Here's how the part is built. I have some questions about the finished solid (model axes, mm). A direction names the side the tool comes from. Give positions to 0.01 mm unless a question says otherwise; leave off trailing zeros. Loops run counter-clockwise (first coordinate to the right, second up) from the corner with the lowest first, then second, coordinate; pieces in that order, holes last. Notation, with made-up numbers: (71.5, 49.5) - (81.5, 49.5) arc R31 cw to (81.5, 86.5) - close; hole circle Ø1 at (-1.5, 14). An arc over 180 degrees is marked (long way). Return JSON: item names as keys, results as strings. Group by question number.
(1) If we section it at D-D (z = -9): Please give me the cut outline in (x, y).
(2) For P1, Ø5.5, axis at x = 7.5, z = -23, coming from the +Y side; P2, Ø6.5, axis at y = 5.5, z = -20.5, coming from the +X side; P3, Ø3, axis at x = 11, z = -17, coming from the -Y side; P4, Ø8, axis at x = 9, z = 15.5, coming from the -Y side, each with a flat end and sliding along its axis, tell me the tip position at first contact or that it passes through.
(3) On a 3-axis mill with a long thin cutter (end or side, diameter ignored), from which of +Z, -Z, +X, -X, +Y, -Y can I reach the whole of each face in a straight line? I mean faces 1 (the flat face through (-9, 12.7, 22)), 2 (the flat face through (14, 16, 6.35)), 3 (the flat face through (14, -3, 6.35)). Say none if no direction works.
(4) If we section it at A-A (y = -0.75): Please give me the cut outline in (x, z).
(5) If we mould it in two halves opening along X, with no side actions, what happens to faces 4 (the flat face through (6.35, 10, 29)), 5 (the flat face through (-12.7, 6, 26)), 6 (the flat face through (-14, -3, -6.35))? For each: released by +X, released by -X, zero draft, split by the parting line, or undercut.
(6) I need wall thicknesses on probe 1 along X at (y, z) = (7.5, 34); probe 2 along Z at (x, y) = (0.5, 10); probe 3 along Y at (x, z) = (7, 12.5). Which ranges of each line are inside material? Lowest first, please. Write a range as [from, to].
(7) If we section it at B-B (y = 7.5): Please give me the cut outline in (x, z).
(8) If we section it at C-C (x = -5.5): Please give me the cut outline in (y, z), then the cut area to 3 significant figures.
```python
from build123d import *
from build123d.topology import SkipClean

# Parameters (mm, degrees)
SKETCH1_R           = 19.05
SKETCH1_R_2         = 12.7
BOSS_EXTRUDE1_DEPTH = 12.7
BOSS_EXTRUDE4_START = -19.05
BOSS_EXTRUDE4_DEPTH = 25.4
BOSS_EXTRUDE7_DEPTH = 12.7
CIRPATTERN3_COUNT   = 2
CIRPATTERN3_ANGLE   = 90
SKETCH14_W          = 12.7
SKETCH14_H          = 19.05
CUT_EXTRUDE1_DEPTH  = 6.35
SKETCH15_R          = 3.175
CUT_EXTRUDE2_DEPTH  = 6.35
CIRPATTERN4_COUNT   = 2


with BuildPart() as part:
    # Sketch1 → Boss-Extrude1 (new body)
    with BuildSketch(Plane(origin=(0, 0, 0), x_dir=(1, 0, 0), z_dir=(0, 1, 0))):
        with Locations(Location((0, 0, 0), (0, 0, 270))):
            Circle(SKETCH1_R)
        with Locations(Location((0, 0, 0), (0, 0, 270))):
            Circle(SKETCH1_R_2, mode=Mode.SUBTRACT)
    extrude(amount=BOSS_EXTRUDE1_DEPTH)

    # Sketch5 → Boss-Extrude4 (add)
    with SkipClean():  # the faces are left unmerged after this step: merging them gives an invalid solid
        with BuildSketch(Plane(origin=(0, 12.7, 0), x_dir=(1, 0, 0), z_dir=(0, 1, 0)).offset(BOSS_EXTRUDE4_START)):
            with BuildLine():
                ThreePointArc((-17.960512, 6.35), (-19.05, 0), (-17.960512, -6.35))
                Line((-17.960512, -6.35), (-10.998523, -6.35))
                ThreePointArc((-10.998523, -6.35), (-12.7, 0), (-10.998523, 6.35))
                Line((-10.998523, 6.35), (-17.960512, 6.35))
            make_face()
            with BuildLine():
                Line((10.998523, -6.35), (17.960512, -6.35))
                ThreePointArc((17.960512, -6.35), (18.775653, -3.221393), (19.05, 0))
                ThreePointArc((19.05, 0), (18.775653, 3.221393), (17.960512, 6.35))
                Line((17.960512, 6.35), (10.998523, 6.35))
                ThreePointArc((10.998523, 6.35), (12.267258, 3.287002), (12.7, 0))
                ThreePointArc((12.7, 0), (12.267258, -3.287002), (10.998523, -6.35))
            make_face()
        boss_extrude4 = extrude(amount=BOSS_EXTRUDE4_DEPTH)

    # Sketch13 → Boss-Extrude7 (add)
    with SkipClean():  # the faces are left unmerged after this step: merging them gives an invalid solid
        with BuildSketch(Plane.XZ):
            with BuildLine():
                ThreePointArc((0, 19.05), (6.797461, 17.795983), (12.7, 14.199032))
                Line((12.7, 14.199032), (12.7, 38.1))
                Line((12.7, 38.1), (-12.7, 38.1))
                Line((-12.7, 38.1), (-12.7, 14.199032))
                ThreePointArc((-12.7, 14.199032), (-6.797461, 17.795983), (0, 19.05))
            make_face()
        boss_extrude7 = extrude(amount=-BOSS_EXTRUDE7_DEPTH)

    # CirPattern3: Boss-Extrude4 ×2 about axis
    with SkipClean():  # the faces are left unmerged after this step: merging them gives an invalid solid
        cirpattern3_axis = Axis((0, 12.7, 0), (0, 1, 0))
        for i in range(1, CIRPATTERN3_COUNT):
            add(boss_extrude4.rotate(cirpattern3_axis, i * CIRPATTERN3_ANGLE / (CIRPATTERN3_COUNT - 1)))

    # Sketch14 → Cut-Extrude1 (cut)
    with SkipClean():  # the faces are left unmerged after this step: merging them gives an invalid solid
        with BuildSketch(Plane(origin=(0, 12.7, 0), x_dir=(1, 0, 0), z_dir=(0, 1, 0))):
            with Locations((0, -28.575)):
                Rectangle(SKETCH14_W, SKETCH14_H)
        cut_extrude1 = extrude(amount=-CUT_EXTRUDE1_DEPTH, mode=Mode.SUBTRACT)

    # Sketch15 → Cut-Extrude2 (cut)
    with SkipClean():  # the faces are left unmerged after this step: merging them gives an invalid solid
        with BuildSketch(Plane(origin=(0, 6.35, 0), x_dir=(1, 0, 0), z_dir=(0, 1, 0))):
            with Locations(Location((0, -28.575, 0), (0, 0, 270))):
                Circle(SKETCH15_R)
        cut_extrude2 = extrude(amount=-CUT_EXTRUDE2_DEPTH, mode=Mode.SUBTRACT)

    # CirPattern4: Boss-Extrude7, Cut-Extrude1, Cut-Extrude2 ×2 about axis
    cirpattern4_axis = Axis((0, 0, 0), (0, 1, 0))
    add([boss_extrude7.rotate(cirpattern4_axis, i * 360 / CIRPATTERN4_COUNT) for i in range(1, CIRPATTERN4_COUNT)])
    add([cut_extrude1.rotate(cirpattern4_axis, i * 360 / CIRPATTERN4_COUNT) for i in range(1, CIRPATTERN4_COUNT)], mode=Mode.SUBTRACT)
    add([cut_extrude2.rotate(cirpattern4_axis, i * 360 / CIRPATTERN4_COUNT) for i in range(1, CIRPATTERN4_COUNT)], mode=Mode.SUBTRACT)


solid = part.part
```
Values:
{
 "1": {"outline": "(-16.79, 0) - (-8.96, 0) - (-8.96, 12.7) - (-16.79, 12.7) - close; (8.96, 0) - (16.79, 0) - (16.79, 12.7) - (8.96, 12.7) - close"},
 "2": {"P1": "y = 12.7", "P2": "x = 12.7", "P3": "y = 0", "P4": "y = -6.35"},
 "3": {"face 1": "+Z, -X, +Y", "face 2": "+Z, +X, -X, +Y", "face 3": "+Z, +X, -X, -Y"},
 "4": {"outline": "(-17.96, -6.35) - (-11, -6.35) arc R12.7 cw to (-11, 6.35) - (-17.96, 6.35) arc R19.05 ccw to start; (-6.35, -17.96) arc R19.05 ccw to (0, -19.05) arc R19.05 ccw to (6.35, -17.96) - (6.35, -11) arc R12.7 cw to (-6.35, -11) - close; (-6.35, 11) arc R12.7 cw to (6.35, 11) - (6.35, 17.96) arc R19.05 ccw to (-6.35, 17.96) - close; (11, -6.35) - (17.96, -6.35) arc R19.05 ccw to (19.05, 0) arc R19.05 ccw to (17.96, 6.35) - (11, 6.35) arc R12.7 cw to start"},
 "5": {"face 4": "undercut", "face 5": "released by -X", "face 6": "zero draft"},
 "6": {"probe 1": "[-12.7, -6.35], [6.35, 12.7]", "probe 2": "[-19.05, -12.69], [12.69, 19.05]", "probe 3": "[0, 12.7]"},
 "7": {"outline": "(-12.7, -38.1) - (-6.35, -38.1) - (-6.35, -19.05) - (6.35, -19.05) - (6.35, -38.1) - (12.7, -38.1) - (12.7, -14.2) arc R19.05 ccw to (17.96, -6.35) arc R19.05 ccw to (19.05, 0) arc R19.05 ccw to (17.96, 6.35) arc R19.05 ccw to (12.7, 14.2) - (12.7, 38.1) - (6.35, 38.1) - (6.35, 19.05) - (-6.35, 19.05) - (-6.35, 38.1) - (-12.7, 38.1) - (-12.7, 14.2) arc R19.05 ccw to (-12.7, -14.2) - close; hole circle Ø25.4 at (0, 0)"},
 "8": {"outline": "(-6.35, -18.24) - (0, -18.24) - (0, -38.1) - (6.35, -38.1) - (6.35, -19.05) - (12.7, -19.05) - (12.7, -18.24) - (19.05, -18.24) - (19.05, -11.45) - (-6.35, -11.45) - close; (-6.35, 11.45) - (19.05, 11.45) - (19.05, 18.24) - (12.7, 18.24) - (12.7, 19.05) - (6.35, 19.05) - (6.35, 38.1) - (0, 38.1) - (0, 18.24) - (-6.35, 18.24) - close", "area": "608 mm2"}
}
